Job drawing, mm, ordinate dimensions from the low corner. One solid piece. Give positions to 0.01 mm unless a question says otherwise; leave off trailing zeros. Loops run counter-clockwise (first coordinate to the right, second up) from the corner with the lowest first, then second, coordinate; pieces in that order, holes last.
Item 1: Saw through at C-C on z = 0.75. Give the number of separate pieces and of enclosed holes in the cut face, plus the area to 3 significant figures.
Item 2: Saw through at A-A on y = 45. Give the cut face in (x, z), plus the area to 3 significant figures.
Item 3: Saw through at B-B on x = 41.5. Give the cut face in (y, z).
Item 4: Probe probe 1 along X at (y, z) = (26, 1.55); probe 2 along Y at (x, z) = (24.5, 2.4). List the from-to ranges inside material, lowest first.
Item 5: Drop flat-ended pins along their axis: P1, Ø0.9, axis at x = 46.5, z = 1, coming from the -Y side; P2, Ø1.5, axis at x = 1, z = 1.5, coming from the -Y side; P3, Ø0.9, axis at y = 64, z = 2, coming from the -X side. Give the stop position or say it passes through.
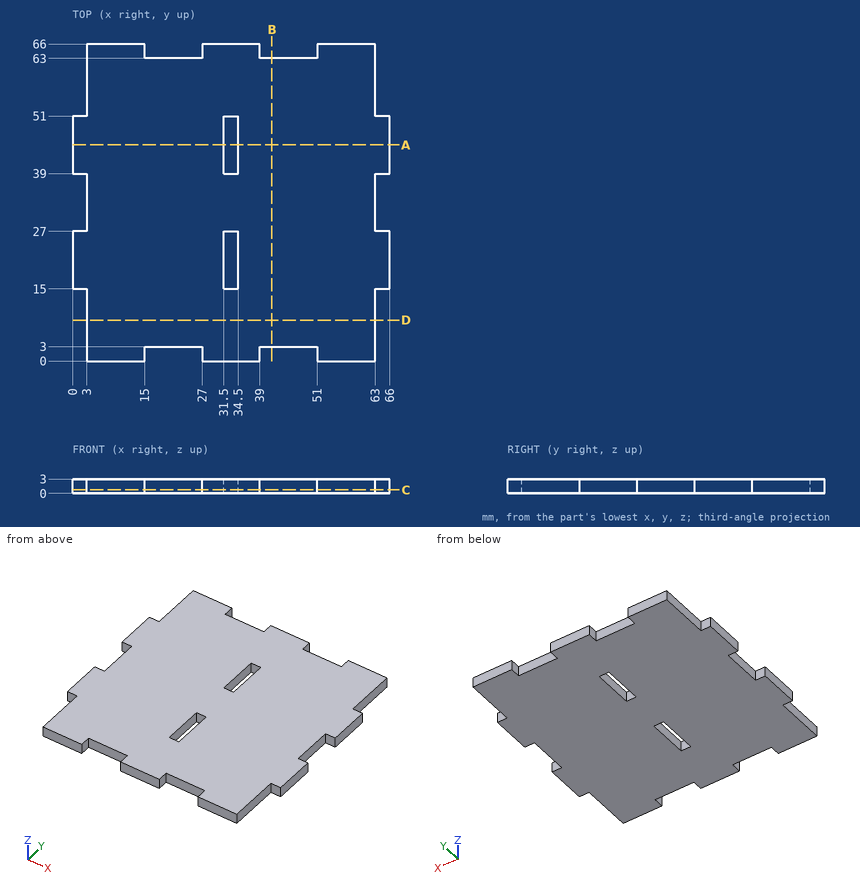
Results below:
1. separate pieces: 1
1. enclosed holes: 2
1. area: 3,890 mm2
2. outline: (0, 0) - (31.5, 0) - (31.5, 3) - (0, 3) - close; (34.5, 0) - (66, 0) - (66, 3) - (34.5, 3) - close
2. area: 189 mm2
3. outline: (3, 0) - (63, 0) - (63, 3) - (3, 3) - close
4. probe 1: x = 0 to 31.5, 34.5 to 66
4. probe 2: y = 3 to 63
5. P1: stops at y = 3
5. P2: stops at y = 15
5. P3: stops at x = 3
